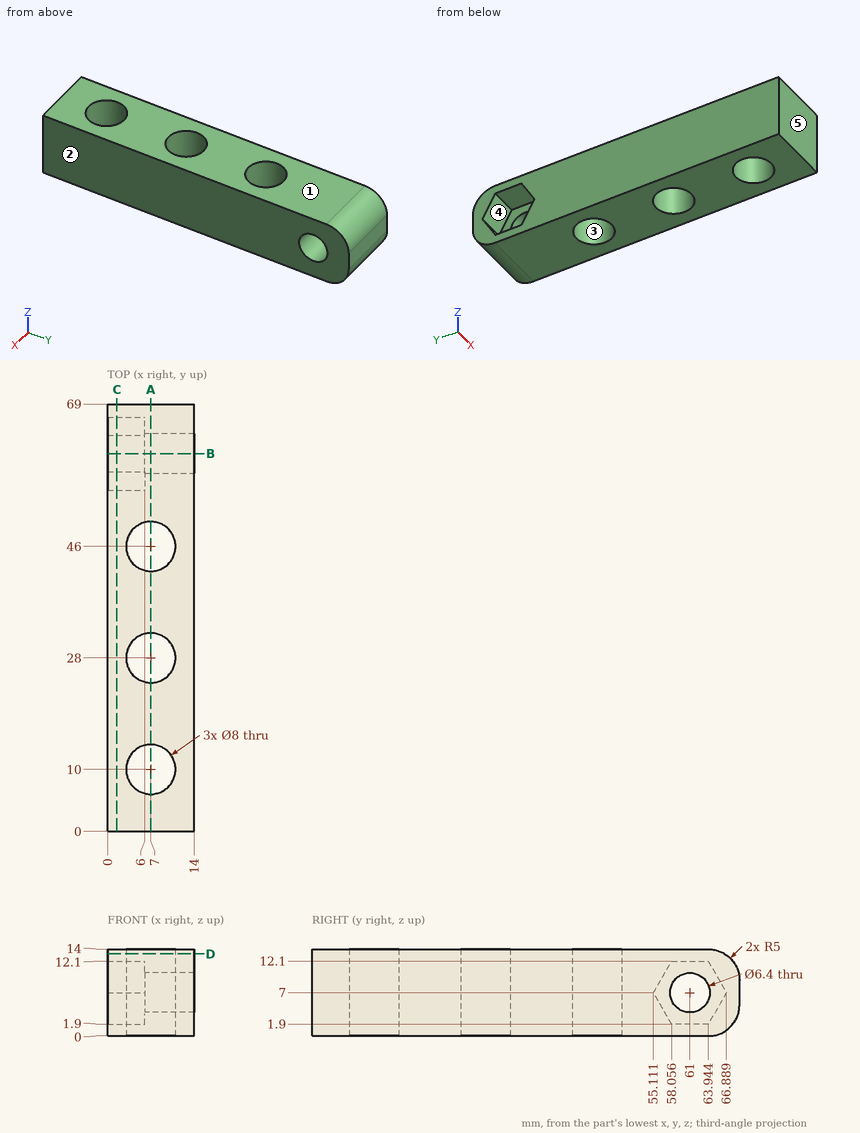
Geometry: see drawing. Coordinates: mm, zero at the bounding-box minimum. A direction names the side the tool comes from. Coordinates: 2 decimals unless noted, no trailing zeros. Loops run counter-clockwise (first coordinate to the right, second up) from the corner with the lowest first, then second, coordinate; pieces in that order, holes last. Notation, with made-up numbers: M 55.25,2 L 100.25,2 A19 cw 100.25,32 Z; hole C 11,65.25 d9. An arc over 180 degrees is marked long. Answer in a Markdown table with one row per item.
1. Section D-D, the plane z = 13.25. Output: boundary loops of the cut face in (x, y), then the cut area to 3 significant figures.
Response:
| item | result |
|---|---|
| outline | M 0,0 L 14,0 L 14,66.63 L 0,66.63 Z; hole C 7,10 d8; hole C 7,28 d8; hole C 7,46 d8 |
| area | 782 mm2 |
2. First-contact query: pin 1 (7 mm diameter, centred on x = 7, y = 28, fed in from +Z). Flat tip, straight axial feed; report the tip coordinate or a pass-through.
Response:
| item | result |
|---|---|
| pin 1 | passes through |
3. Draft query along X for the marked faces 1, 2 and 3. Return one class per face: pulls with the +X half, pulls with the -X half, needs draft (parallel to the pull), parting line crosses it, or undercut.
Response:
| item | result |
|---|---|
| face 1 | needs draft |
| face 2 | pulls with the +X half |
| face 3 | undercut |
4. Section B-B, the plane y = 61. Output: boundary loops of the cut face in (x, z).
Response:
| item | result |
|---|---|
| outline | M 0,0 L 14,0 L 14,3.8 L 6,3.8 L 6,1.9 L 0,1.9 Z; M 0,12.1 L 6,12.1 L 6,10.2 L 14,10.2 L 14,14 L 0,14 Z |
5. Section A-A, the plane x = 7. Output: boundary loops of the cut face in (y, z).
Response:
| item | result |
|---|---|
| outline | M 0,0 L 6,0 L 6,14 L 0,14 Z; M 14,0 L 24,0 L 24,14 L 14,14 Z; M 32,0 L 42,0 L 42,14 L 32,14 Z; M 50,0 L 64,0 A5 ccw 69,5 L 69,9 A5 ccw 64,14 L 50,14 Z; hole C 61,7 d6.4 |
6. Reachability of the marked faces 4 and 5 from +Z, -Z, +X, -X, +Y, -Y: full face, straight path, thin tool, end or side. Return the list, or none.
Response:
| item | result |
|---|---|
| face 4 | -X |
| face 5 | +Z, -Z, +X, -X, -Y |
7. Material intervals for line 1 (Y direction, x = 7, z = 9); line 2 (Y direction, x = 4.25, z = 3.75) (1 decimal); line 3 (Y direction, x = 7, z = 10.25), sorted ascending.
Response:
| item | result |
|---|---|
| line 1 | y = 0 to 6, 14 to 24, 32 to 42, 50 to 58.5, 63.5 to 69 |
| line 2 | y = 0 to 7.1, 12.9 to 25.1, 30.9 to 43.1, 48.9 to 57, 65 to 68.8 |
| line 3 | y = 0 to 6, 14 to 24, 32 to 42, 50 to 68.84 |
8. Section C-C, the plane x = 1.5. Output: boundary loops of the cut face in (y, z) (1 decimal), then the cut area to 3 significant figures.
Response:
| item | result |
|---|---|
| outline | M 0,0 L 64,0 A5 ccw 69,5 L 69,9 A5 ccw 64,14 L 0,14 Z; hole M 55.1,7 L 58.1,1.9 L 63.9,1.9 L 66.9,7 L 63.9,12.1 L 58.1,12.1 Z |
| area | 865 mm2 |
